Design review of the part built by this model. Coordinates are the model's own, in mm. Face numbers are marked on the shaded views. Coordinates: 2 decimals unless noted, no trailing zeros. Order: outer loops, then holes, each group sorted by start corner. A loop starts at its lowest first (then second) coordinate and runs counter-clockwise, first axis right, second up. Notation, with made-up numbers: M 84.25,79 L 112.25,79 A21 cw 112.25,111 Z; hole C 61.5,53.25 d1. An arc over 180 degrees is marked long. Answer in a Markdown table with one row per item.
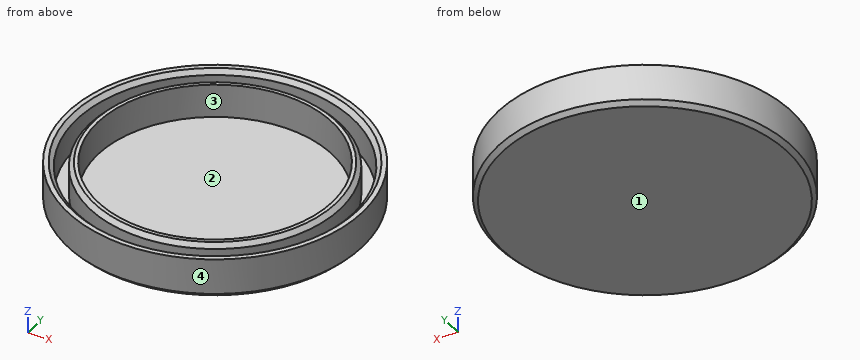
from build123d import *

# Parameters (mm, degrees)
F0_R     = 44
F1_DEPTH = 2
F2_R     = 44
F2_R_2   = 41.25
F2_R_3   = 37.4
F2_R_4   = 35
F3_DEPTH = 10
F4_SIZE  = 1.3


with BuildPart() as f1:
    # F0 (on Top) → F1 (new body)
    with BuildSketch(Plane.XY):
        Circle(F0_R)
    extrude(amount=F1_DEPTH)

    # F2 (on face) → F3 (join)
    with BuildSketch(Plane.XY.offset(2)):
        Circle(F2_R)
        Circle(F2_R_2, mode=Mode.SUBTRACT)
        Circle(F2_R_3)
        Circle(F2_R_4, mode=Mode.SUBTRACT)
    extrude(amount=F3_DEPTH)

    # F4
    f4_edges = [f1.edges().sort_by_distance(p)[0] for p in [
        (-41.25, 0, 12),
        (-37.4, 0, 12),
        (-44, 0, 0),
    ]]
    chamfer(f4_edges, length=F4_SIZE)


solid = f1.part
(1) Draft analysis for pull direction Y (two halves, no side actions). For the marked faces 1, 2, 3 and 4, state which applies: pulls with the +Y half, pulls with the -Y half, needs draft (parallel to the pull), parting line crosses it, or undercut.
Return value:
| item | result |
|---|---|
| face 1 | needs draft |
| face 2 | undercut |
| face 3 | undercut |
| face 4 | parting line crosses it |
(2) Add section A-A, the plane y = 0. Give the boundary of the cut face in (x, z), and give its area (3 significant figures).
Return value:
| item | result |
|---|---|
| outline | M -44,1.3 L -42.7,0 L 42.7,0 L 44,1.3 L 44,12 L 42.55,12 L 41.25,10.7 L 41.25,2 L 37.4,2 L 37.4,10.7 L 36.1,12 L 35,12 L 35,2 L -35,2 L -35,12 L -36.1,12 L -37.4,10.7 L -37.4,2 L -41.25,2 L -41.25,10.7 L -42.55,12 L -44,12 Z |
| area | 274 mm2 |
(3) Add section B-B, the plane z = 7.75. Give the boundary of the cut face in (x, y).
Return value:
| item | result |
|---|---|
| outline | C 0,0 d88; C 0,0 d74.8; hole C 0,0 d82.5; hole C 0,0 d70 |
(4) Insertion check: pin 1 Ø6 at (x, z) = (-32.5, 2) entering from -Y; pin 2 Ø1.5 at (x, z) = (-6.5, 3.5) entering from +Y; pin 3 Ø2 at (x, y) = (22.5, -23) entering from +Z. Each pin has a flat end and moves straight along its axis. Give the tip position at first contact, or say it passes through.
Return value:
| item | result |
|---|---|
| pin 1 | stops at y = -32.65 |
| pin 2 | stops at y = 43.62 |
| pin 3 | stops at z = 2 |
(5) For line 1 along Y through (x, z) = (0, 6.5); line 2 along Y through (x, z) = (30.5, 2.5); line 3 along X through (y, z) = (-23, 11), list the stretches that pass through material, from the lowest coordinate up. Write a range as from..to.
Return value:
| item | result |
|---|---|
| line 1 | y = -44..-41.25, -37.4..-35, 35..37.4, 41.25..44 |
| line 2 | y = -31.71..-27.77, -21.65..-17.17, 17.17..21.65, 27.77..31.71 |
| line 3 | x = -37.51..-34.6, -29.11..-26.38, 26.38..29.11, 34.6..37.51 |
